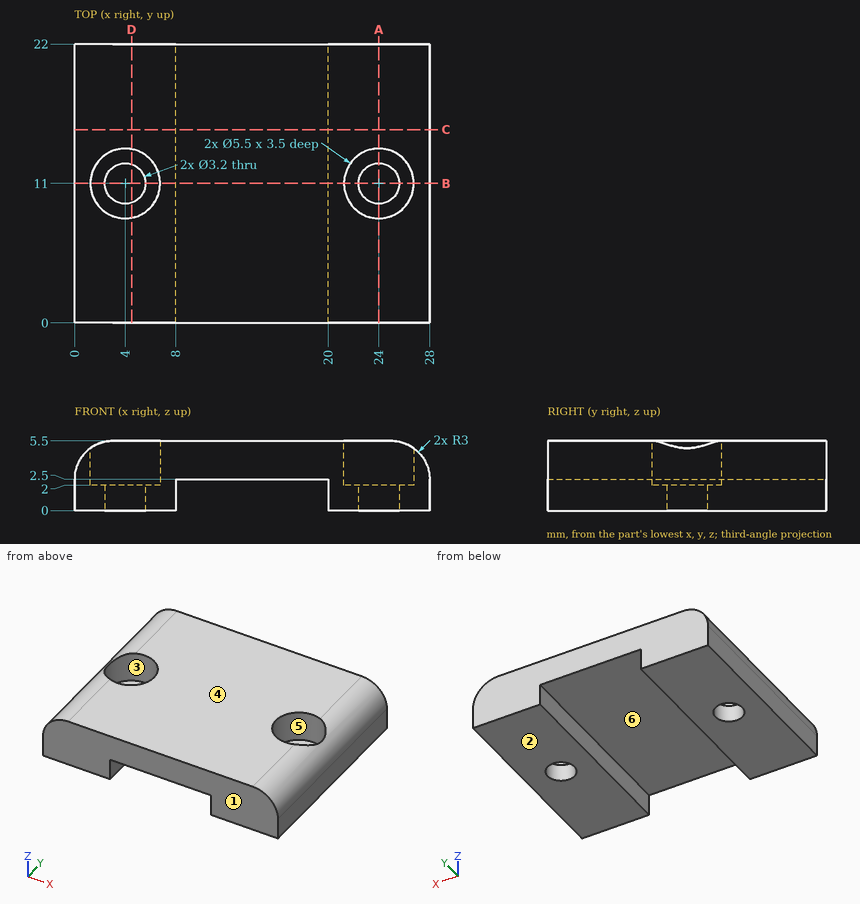
The drawing under review shows one solid part. Ordinate dimensions are in mm from its lowest x, y, z. A direction names the side the tool comes from. Round coordinates to 2 decimals unless told otherwise and drop trailing zeros. Loops run counter-clockwise (first coordinate to the right, second up) from the corner with the lowest first, then second, coordinate; pieces in that order, holes last. Notation, with made-up numbers: (39, 9) - (98, 9) arc R36 ccw to (98, 43) - close; hole circle Ø4 at (-9.5, 18.5). An arc over 180 degrees is marked (long way). Use one line per item in the form item = value.
Item 1: Consider section A-A on x = 24. Write out the cut boundary in (y, z).
Answers:
outline = (0, 0) - (9.4, 0) - (9.4, 2) - (8.25, 2) - (8.25, 5.5) - (0, 5.5) - close; (12.6, 0) - (22, 0) - (22, 5.5) - (13.75, 5.5) - (13.75, 2) - (12.6, 2) - close
Item 2: Consider section B-B on y = 11. Write out the cut boundary in (x, z), then the cut area to 3 significant figures.
Answers:
outline = (0, 0) - (2.4, 0) - (2.4, 2) - (1.25, 2) - (1.25, 4.94) arc R3 ccw to (0, 2.5) - close; (5.6, 0) - (8, 0) - (8, 2.5) - (20, 2.5) - (20, 0) - (22.4, 0) - (22.4, 2) - (21.25, 2) - (21.25, 5.5) - (6.75, 5.5) - (6.75, 2) - (5.6, 2) - close; (25.6, 0) - (28, 0) - (28, 2.5) arc R3 ccw to (26.75, 4.94) - (26.75, 2) - (25.6, 2) - close
area = 69.5 mm^2
Item 3: For line 1 (X direction, y = 20, z = 1.85); line 2 (Y direction, x = 24, z = 2.9); line 3 (X direction, y = 10.5, z = 2.9), list the stretches that pass through material, from the lowest coordinate up.
Answers:
line_1 = 0 to 8, 20 to 28
line_2 = 0 to 8.25, 13.75 to 22
line_3 = 0.03 to 1.3, 6.7 to 21.3, 26.7 to 27.97
Item 4: Consider section C-C on y = 15.25. Write out the cut boundary in (x, z), then the cut area to 3 significant figures.
Answers:
outline = (0, 0) - (8, 0) - (8, 2.5) - (20, 2.5) - (20, 0) - (28, 0) - (28, 2.5) arc R3 ccw to (25, 5.5) - (3, 5.5) arc R3 ccw to (0, 2.5) - close
area = 120 mm^2
Item 5: Consider section D-D on x = 4.5. Write out the cut boundary in (y, z), then the cut area to 3 significant figures.
Answers:
outline = (0, 0) - (9.48, 0) - (9.48, 2) - (8.3, 2) - (8.3, 5.5) - (0, 5.5) - close; (12.52, 0) - (22, 0) - (22, 5.5) - (13.7, 5.5) - (13.7, 2) - (12.52, 2) - close
area = 96.0 mm^2
Item 6: Clearance check with flat-ended pins moving along their axes: P1, Ø1.6, axis at x = 24, y = 10, coming from the +Z side; P2, Ø1, axis at x = 18, y = 6, coming from the -Z side. State where each tip first meets the part, or that it passes through.
Answers:
P1 = 2
P2 = 2.5
Item 7: Tool access review of the marked faces 4, 5 and 6: name each direction out of +Z, -Z, +X, -X, +Y, -Y from which nothing blocks a thin tool from reaching the whole face with its end or side.
Answers:
face_4 = +Z, +X, -X, +Y, -Y
face_5 = +Z
face_6 = -Z, +Y, -Y
Item 8: Mouldability with a two-part tool opening along Y and no side actions: class the marked faces 1, 2 and 3 as +Y half, -Y half, draft (parallel to the pull), parting line (faces both ways), or undercut.
Answers:
face_1 = -Y half
face_2 = draft
face_3 = undercut
